Source: CAD feature listing. Evaluate the final solid. Frame: model axes, mm. A direction names the side the tool comes from. Round coordinates to 2 decimals unless told otherwise and drop trailing zeros. Write each loop counter-clockwise with the first axis right and the second up, starting at its lowest first coordinate (ties: lowest second). Pieces come first, ordered by that corner, then holes. Notation, with made-up numbers: (88, 76.5) -> (126, 76.5) arc R26 cw to (126, 93.5) -> close; hole circle Ø5 at (62.5, -36.5). An arc over 180 degrees is marked (long way). Put each result on its own line as item: value.
Autodesk Inventor part; units mm, degrees
ref_plane "Work Plane2" through (-7, 76.75, -10.5439) normal (0, 0, 1) x (1, 0, 0)
ref_plane "YZ Plane" through (0, 0, 0) normal (1, 0, 0) x (0, 1, 0)
ref_plane "XZ Plane" through (0, 0, 0) normal (0, 1, 0) x (-1, 0, 0)
ref_plane "Work Plane1" through (0, 0, 0) normal (0, 0, 1) x (1, 0, 0)
sketch "Sketch1" plane through (0, 0, 0) normal (0, 0, 1) x (1, 0, 0)
  circle A0 centre (11, 82.9899) radius 1.6
  circle A1 centre (-3, 82.9899) radius 1.6
  circle A2 centre (7.5, 24) radius 6.4506
  circle A3 centre (7.5, 64) radius 6.4305
  arc A4 (0, 42.6389) -> (0, 45.3611) centre (-0.5, 44) ccw
  line L0 (0, -32) -> (0, 42.6389)
  line L1 (0, -32) -> (15, -32)
  line L2 (15, 35.9533) -> (15, -32)
  arc A5 (15, 35.9533) -> (15, 52.0467) centre (7.5, 44) ccw
  line L3 (15, 52.0467) -> (15, 86)
  line L4 (0, 45.3611) -> (0, 74)
  circle A6 centre (7.5, 36) radius 1.45
  circle A7 centre (7.5, 52) radius 1.45
  circle A8 centre (15.5, 44) radius 1.45
  circle A9 centre (7.5, 44) radius 6
  line L5 (-6.6903, 74) -> (15, 74)
  line L6 (15, 74) -> (15, 107.8848)
  line L7 (15, 107.8848) -> (-6.6903, 107.8848)
  line L8 (-6.6903, 107.8848) -> (-6.6903, 74)
  line L9 (15, 86) -> (-7, 86)
  line L10 (-7, 86) -> (-7, 74)
  line L11 (-7, 74) -> (0, 74)
  point P0 (0, 0)
extrude "Extrusion1" add sketch "Sketch1" along normal blind 4 contours L5 L8 L9 L3 | L8 L7 L6 L9
sketch "Sketch2" plane through (0, 0, 0) normal (0, 0, -1) x (-1, 0, 0)
  circle A0 centre (3, 82.9899) radius 1.6
  circle A1 centre (-11, 82.9899) radius 1.6
  line L0 (6.6903, 74) -> (6.6903, 107.8848)
  line L1 (6.6903, 107.8848) -> (-15, 107.8848)
  line L2 (-15, 107.8848) -> (-15, 74)
  line L3 (-15, 74) -> (6.6903, 74)
  line L4 (-15, 74) -> (-15, 107.8848)
  line L5 (-15, 107.8848) -> (6.6903, 107.8848)
  line L6 (6.6903, 107.8848) -> (6.6903, 87.9676)
  line L7 (6.6903, 87.9676) -> (-15, 87.9676)
  line L8 (-15, 87.9676) -> (-15, 107.8848)
  point P0 (0, 0)
ref_plane "Work Plane2" through (-7, 76.75, -10.5439) normal (0, 0, 1) x (1, 0, 0)
extrude "Extrusion2" add sketch "Sketch2" along normal up to surface (10.5439 mm away) contours L7 L2 L1 L0
sketch "Sketch3" plane through (15, 87.9676, -10.5439) normal (0, 0, -1) x (-1, 0, 0)
  line L0 (0, 19.9172) -> (0, 0)
  line L1 (0, 0) -> (21.6903, 0)
  line L2 (21.6903, 0) -> (21.6903, 19.9172)
  line L3 (21.6903, 19.9172) -> (0, 19.9172)
  line L4 (0, 19.9172) -> (21.6903, 19.9172)
  line L5 (0, -13.9676) -> (0, 19.9172)
  line L6 (21.6903, 19.9172) -> (0, 19.9172)
  line L7 (0, 19.9172) -> (0, 14.7562)
  line L8 (0, 14.7562) -> (21.6903, 14.7562)
  line L9 (21.6903, 14.7562) -> (21.6903, 19.9172)
  line L10 (21.6903, 0) -> (21.6903, 19.9172)
  line L11 (0, 19.9172) -> (0, 0)
  line L12 (21.6903, 19.9172) -> (0, 19.9172)
  line L13 (0, 19.9172) -> (0, 14.63)
  line L14 (0, 14.63) -> (21.6903, 14.63)
  line L15 (21.6903, 14.63) -> (21.6903, 19.9172)
  line L16 (22, 14.2824) -> (14.4, 14.2824)
  point P0 (15, -87.9676)
extrude "Extrusion3" add sketch "Sketch3" along normal blind 6 contours L3 L2 L8 L0
sketch "Sketch4" plane through (-6.6903, 74, 4) normal (-1, 0, 0) x (0, 0, 1)
  circle A0 centre (-28.5439, 14.25) radius 10.8
  line L0 (-20.5439, 33.8848) -> (-20.5439, 28.7239)
  line L1 (0, 0) -> (-20.5439, 0)
  line L2 (-20.5439, 0) -> (-20.5439, 33.8848)
  line L3 (-20.5439, 33.8848) -> (0, 33.8848)
  line L4 (0, 33.8848) -> (0, 0)
  circle A1 centre (-17.0439, 25.75) radius 1.1
  line L5 (-14.5439, 25.75) -> (-14.5439, 2.75)
  arc A2 (-14.5439, 25.75) -> (-17.0439, 28.25) centre (-17.0439, 25.75) ccw
  line L6 (-40.0439, 28.25) -> (-17.0439, 28.25)
  arc A3 (-40.0439, 28.25) -> (-42.5439, 25.75) centre (-40.0439, 25.75) ccw
  line L7 (-42.5439, 2.75) -> (-42.5439, 25.75)
  arc A4 (-42.5439, 2.75) -> (-40.0439, 0.25) centre (-40.0439, 2.75) ccw
  line L8 (-17.0439, 0.25) -> (-40.0439, 0.25)
  arc A5 (-17.0439, 0.25) -> (-14.5439, 2.75) centre (-17.0439, 2.75) ccw
  circle A6 centre (-28.5439, 14.25) radius 11
  circle A7 centre (-40.0439, 25.75) radius 1.025
  circle A8 centre (-17.0439, 25.75) radius 1.025
  circle A9 centre (-17.0439, 2.75) radius 1.025
  circle A10 centre (-40.0439, 2.75) radius 1.025
  line L9 (0, 33.8848) -> (0, 0)
  point P0 (-4, -74)
extrude "Extrusion4" add sketch "Sketch4" along normal blind 2 contours A0 L2 | A0 L2 A6 | L2 L6 A2 L5 A5 L8 A6 | L2 L0 L3 L4 L1 L8 A5 L5 A2 L6 picked at (-19.7185, 15.1251) picked at (-18.4698, 18.1768)
sketch "Sketch5" plane through (-8.6903, 74, 4) normal (-1, 0, 0) x (0, 0, 1)
  circle A0 centre (-28.5439, 14.25) radius 11
  circle A1 centre (-28.5439, 14.25) radius 11.9547
  point P0 (-4, -74)
extrude "Extrusion5" cut sketch "Sketch5" against normal blind 2 contours A0 | A1
chamfer "Chamfer1" distance 10 angle 65 1 edges at (3.1548, 107.8848, 4) measured on face at (7.1032, 107.8848, -2.848)
properties part number "OPENTRONS_Autofocus_NEMA_holder_tmp"
Q1. Cut plane C-C on x = 8.25. Output: boundary loops of the cut face in (y, z), and give its area (3 significant figures).
Ans:
outline: (74, 0) -> (87.97, 0) -> (87.97, -10.54) -> (102.72, -10.54) -> (102.72, -16.54) -> (107.88, -16.54) -> (107.88, -6) -> (86.44, 4) -> (74, 4) -> close
area: 269 mm^2
Q2. Material intervals for line 1 (Z direction, x = -8.2, y = 76.75); line 2 (Y direction, x = -4, z = 1); line 3 (Z direction, x = 2, y = 98), sorted ascending. Write a range as [from, to].
Ans:
line 1: z = [-16.54, -14.07], [-12.02, 4]
line 2: y = [74, 81.74], [84.24, 92.87]
line 3: z = [-10.54, -1.39]
Q3. Draft query along X for faces 1 (the flat face through (-8.69, 91, -6)), 2 (the cylindrical face through (-2.26, 84.41, 1.97)), 3 (the flat face through (-8, 77, -16.544)), 4 (the flat face through (15, 94, -5)). Return one class per face: +X half, -X half, draft (parallel to the pull), parting line (faces both ways), or undercut.
Ans:
face 1: -X half
face 2: undercut
face 3: draft
face 4: +X half
Q4. Cut plane D-D on y = 83.5. Output: boundary loops of the cut face in (x, z), and give its area (3 significant figures).
Ans:
outline: (-8.69, -13.57) -> (-6.69, -13.57) -> (-6.69, 0) -> (-4.52, 0) -> (-4.52, 4) -> (-8.69, 4) -> close; (-1.48, 0) -> (9.48, 0) -> (9.48, 4) -> (-1.48, 4) -> close; (12.52, 0) -> (15, 0) -> (15, 4) -> (12.52, 4) -> close
area: 97.6 mm^2
Q5. Cut plane A-A on y = 76.75. Output: boundary loops of the cut face in (x, z).
Ans:
outline: (-8.69, -16.54) -> (-6.69, -16.54) -> (-6.69, -14.07) -> (-8.69, -14.07) -> close; (-8.69, -12.02) -> (-6.69, -12.02) -> (-6.69, 0) -> (15, 0) -> (15, 4) -> (-8.69, 4) -> close
Q6. Pin query (flat end, axial travel): pin 1 (1.8 mm diameter, centred on x = 5, z = -14, fed in from -Y); pin 2 (1.2 mm diameter, centred on y = 76.75, z = -13.04, fed in from -X); pin 3 (4.5 mm diameter, centred on x = 8, y = 93, fed in from -Z); pin 4 (5 mm diameter, centred on x = 11, y = 82.99, fed in from -Z). Return the tip coordinate at first contact, or that it passes through.
Ans:
pin 1: stops at y = 102.72
pin 2: passes through
pin 3: stops at z = -10.54
pin 4: stops at z = 0
Q7. Cut plane B-B on x = -3. Output: boundary loops of the cut face in (y, z).
Ans:
outline: (74, 0) -> (81.39, 0) -> (81.39, 4) -> (74, 4) -> close; (84.59, 0) -> (87.97, 0) -> (87.97, -10.54) -> (102.72, -10.54) -> (102.72, -16.54) -> (107.88, -16.54) -> (107.88, -6) -> (86.44, 4) -> (84.59, 4) -> close
Q8. Reachability of faces 5 (the cylindrical face through (-7.7, 88.11, -12.59)), 6 (the flat face through (4, 95, -10.544)) from +Z, -Z, +X, -X, +Y, -Y: full face, straight path, thin tool, end or side. Return the list, or none.
Ans:
face 5: -Z, +X, -X
face 6: -Z, +X, -Y
